Verification items for the finished model (mm, model axes). Face numbers are marked on the shaded views. Round coordinates to 2 decimals unless told otherwise and drop trailing zeros. Loops run counter-clockwise (first coordinate to the right, second up) from the corner with the lowest first, then second, coordinate; pieces in that order, holes last. Notation, with made-up numbers: (57.5, 71.5) -> (116.5, 71.5) arc R18 ccw to (116.5, 87.5) -> close; hole circle Ø10 at (57.5, -35.5). An arc over 180 degrees is marked (long way). Use a Markdown table: item, result. Add a question column.
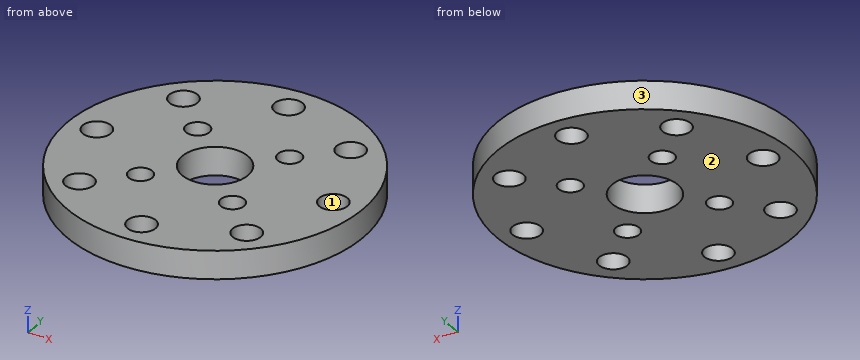
```python
from build123d import *

# Parameters (mm, degrees)
MODEL_R                 = 15.73
MODEL_R_2               = 1.5
MODEL_R_3               = 1.25
MODEL_R_4               = 3.5
SALIENTE_EXTRUIR1_DEPTH = 3


with BuildPart() as part:
    # Model → Saliente-Extruir1 (new body)
    with BuildSketch(Plane.XY):
        with Locations((20.246400491, 284.547476206)):
            Circle(MODEL_R)
        with Locations((20.246400491, 297.275398267)):
            Circle(MODEL_R_2, mode=Mode.SUBTRACT)
        with Locations((7.51847843, 284.547476206)):
            Circle(MODEL_R_2, mode=Mode.SUBTRACT)
        with Locations((20.246400491, 271.819554144)):
            Circle(MODEL_R_2, mode=Mode.SUBTRACT)
        with Locations((32.974322552, 284.547476206)):
            Circle(MODEL_R_2, mode=Mode.SUBTRACT)
        with Locations((15.296653023, 289.497223674)):
            Circle(MODEL_R_3, mode=Mode.SUBTRACT)
        with Locations((15.296653023, 279.597728738)):
            Circle(MODEL_R_3, mode=Mode.SUBTRACT)
        with Locations((25.196147959, 279.597728738)):
            Circle(MODEL_R_3, mode=Mode.SUBTRACT)
        with Locations((25.196147959, 289.497223674)):
            Circle(MODEL_R_3, mode=Mode.SUBTRACT)
        with Locations((20.246400491, 284.547476206)):
            Circle(MODEL_R_4, mode=Mode.SUBTRACT)
        with Locations((11.246400491, 293.547476206)):
            Circle(MODEL_R_2, mode=Mode.SUBTRACT)
        with Locations((11.246400491, 275.547476206)):
            Circle(MODEL_R_2, mode=Mode.SUBTRACT)
        with Locations((29.246400491, 275.547476206)):
            Circle(MODEL_R_2, mode=Mode.SUBTRACT)
        with Locations((29.246400491, 293.547476206)):
            Circle(MODEL_R_2, mode=Mode.SUBTRACT)
    extrude(amount=SALIENTE_EXTRUIR1_DEPTH)


solid = part.part
```
1) Sectioned sample at D-D on y = 287. Enter the section's corners in (x, z), then the cut area to 3 significant figures.
2) Sectioned sample at C-C on z = 2.6. State how many separate pieces and enclosed holes the cut face has, then the cut area to 3 significant figures.
3) Sectioned sample at A-A on y = 279. Enter the section's corners in (x, z).
4) Sectioned sample at B-B on x = 12. Enter the section's corners in (y, z), then the cut area to 3 significant figures.
5) Release check for a two-part mould opening along X. For the marked faces 1, 2 and 3 record: released by +X, released by -X, zero draft, split by the parting line, or undercut.
6) Go/stop test with a flat-tipped pin: pin 1 (1.5 mm diameter, centred on x = 16, z = 1.5, fed in from +Y). Record where the tip stops, or that it passes through.
7) Thickness scan on line 1 (X direction, y = 284.5, z = 0.8); line 2 (X direction, y = 290.5, z = 2.05); line 3 (Y direction, x = 26, z = 1.85). Record the ranges inside material, lowest first.
Geometry results:
| question | item | result |
|---|---|---|
| 1 | outline | (4.71, 0) -> (17.75, 0) -> (17.75, 3) -> (4.71, 3) -> close; (22.74, 0) -> (35.78, 0) -> (35.78, 3) -> (22.74, 3) -> close |
| 1 | area | 78.2 mm^2 |
| 2 | separate pieces | 1 |
| 2 | enclosed holes | 13 |
| 2 | area | 663 mm^2 |
| 3 | outline | (5.53, 0) -> (14.2, 0) -> (14.2, 3) -> (5.53, 3) -> close; (16.39, 0) -> (24.1, 0) -> (24.1, 3) -> (16.39, 3) -> close; (26.29, 0) -> (34.97, 0) -> (34.97, 3) -> (26.29, 3) -> close |
| 4 | outline | (271.15, 0) -> (274.25, 0) -> (274.25, 3) -> (271.15, 3) -> close; (276.84, 0) -> (292.25, 0) -> (292.25, 3) -> (276.84, 3) -> close; (294.84, 0) -> (297.94, 0) -> (297.94, 3) -> (294.84, 3) -> close |
| 4 | area | 64.8 mm^2 |
| 5 | face 1 | undercut |
| 5 | face 2 | zero draft |
| 5 | face 3 | split by the parting line |
| 6 | pin 1 | y = 299.88 |
| 7 | line 1 | 4.52 to 6.02, 9.02 to 16.75, 23.75 to 31.48, 34.47 to 35.98 |
| 7 | line 2 | 5.69 to 14.55, 16.04 to 24.45, 25.94 to 34.81 |
| 7 | line 3 | 269.91 to 278.64, 280.55 to 288.54, 290.45 to 299.19 |
